Verification items for the finished model (mm, model axes). Face numbers are marked on the shaded views. Give positions to 0.01 mm unless a question says otherwise; leave off trailing zeros. Write each loop counter-clockwise with the first axis right and the second up, starting at its lowest first coordinate (ties: lowest second). Pieces come first, ordered by that corner, then holes.
from build123d import *

# Parameters (mm, degrees)
SKETCH1_W           = 188.724999994
SKETCH1_H           = 19.05
BOSS_EXTRUDE1_DEPTH = 109.3
HOLE1_D             = 3.175
HOLE1_DEPTH         = 31.75
HOLE1_CSINK_D       = 10.16
HOLE1_CSINK_ANGLE   = 82
HOLE1_TIP           = 0.953866233
HOLE2_D             = 3.175
HOLE2_DEPTH         = 31.75
HOLE2_CSINK_D       = 10.16
HOLE2_CSINK_ANGLE   = 82
HOLE2_TIP           = 0.953866233
HOLE3_D             = 3.175
HOLE3_DEPTH         = 31.75
HOLE3_CSINK_D       = 10.16
HOLE3_CSINK_ANGLE   = 82
HOLE3_TIP           = 0.953866233
HOLE4_D             = 63.5
HOLE4_DEPTH         = 19.05


with BuildPart() as part:
    # Sketch1 → Boss-Extrude1 (new body)
    with BuildSketch(Plane.XY):
        with Locations((-227.891965966, -292.321060846)):
            Rectangle(SKETCH1_W, SKETCH1_H)
    extrude(amount=BOSS_EXTRUDE1_DEPTH)

    # Hole1
    with Locations(Plane(origin=(-124.004465969, 10.424290059, -12.7), x_dir=(1, 0, 0), z_dir=(0, 0, -1))):
        with Locations((113.649999994, 128.807623392), (113.649999994, 23.940956725), (-94.599999994, 161.374290059), (94.599999994, 161.374290059), (0, 161.374290059), (0, 193.124290059), (0, 440.553783621), (0, 301.970350905), (40.979166666, 301.970350905), (166.795833328, 301.970350905), (207.774999994, 440.553783621), (207.774999994, 333.02141023), (207.774999994, 225.48903684), (207.774999994, 137.424290059), (207.774999994, 10.424290059), (-207.774999994, 10.424290059), (-207.774999994, 137.424290059), (-207.774999994, 225.48903684), (-207.774999994, 333.02141023), (-207.774999994, 440.553783621), (-166.795833328, 301.970350905), (-40.979166666, 301.970350905), (-113.649999994, 23.940956725), (-113.649999994, 128.807623392)):
            CounterSinkHole(HOLE1_D / 2, HOLE1_CSINK_D / 2, depth=HOLE1_DEPTH, counter_sink_angle=HOLE1_CSINK_ANGLE)
            with Locations((0, 0, -(HOLE1_DEPTH + HOLE1_TIP / 2))):  # 118° drill point
                Cone(0, HOLE1_D / 2, HOLE1_TIP, mode=Mode.SUBTRACT)

    # Hole2
    with Locations(Plane(origin=(-124.004465969, 10.424290059, 122), x_dir=(-1, 0, 0), z_dir=(0, 0, 1))):
        with Locations((113.649999994, 128.807623392), (113.649999994, 23.940956725), (-94.599999994, 161.374290059), (94.599999994, 161.374290059), (0, 161.374290059), (0, 193.124290059), (0, 440.553783621), (0, 301.970350905), (40.979166666, 301.970350905), (166.795833328, 301.970350905), (207.774999994, 440.553783621), (207.774999994, 333.02141023), (207.774999994, 225.48903684), (207.774999994, 137.424290059), (207.774999994, 10.424290059), (-207.774999994, 10.424290059), (-207.774999994, 137.424290059), (-207.774999994, 225.48903684), (-207.774999994, 333.02141023), (-207.774999994, 440.553783621), (-166.795833328, 301.970350905), (-40.979166666, 301.970350905), (-113.649999994, 23.940956725), (-113.649999994, 128.807623392)):
            CounterSinkHole(HOLE2_D / 2, HOLE2_CSINK_D / 2, depth=HOLE2_DEPTH, counter_sink_angle=HOLE2_CSINK_ANGLE)
            with Locations((0, 0, -(HOLE2_DEPTH + HOLE2_TIP / 2))):  # 118° drill point
                Cone(0, HOLE2_D / 2, HOLE2_TIP, mode=Mode.SUBTRACT)

    # Hole3
    with Locations(Plane(origin=(-124.004465969, 10.424290059, 122), x_dir=(-1, 0, 0), z_dir=(0, 0, 1))):
        with Locations((-207.774999994, 333.02141023), (-207.774999994, 225.48903684), (-207.774999994, 137.424290059), (-172.166666661, 4.074290059), (-146.083333327, 4.074290059), (-94.599999994, 161.374290059), (0, 161.374290059), (94.599999994, 161.374290059), (146.083333327, 4.074290059), (172.166666661, 4.074290059), (207.774999994, 137.424290059), (207.774999994, 225.48903684), (207.774999994, 333.02141023), (166.795833328, 301.970350905), (40.979166666, 301.970350905), (-40.979166666, 301.970350905), (-166.795833328, 301.970350905), (0, 193.124290059), (0, 301.970350905), (0, 412.366411751), (-126.349999994, 106.824290059), (-126.349999994, 58.624290059), (126.349999994, 58.624290059), (126.349999994, 106.824290059)):
            CounterSinkHole(HOLE3_D / 2, HOLE3_CSINK_D / 2, depth=HOLE3_DEPTH, counter_sink_angle=HOLE3_CSINK_ANGLE)
            with Locations((0, 0, -(HOLE3_DEPTH + HOLE3_TIP / 2))):  # 118° drill point
                Cone(0, HOLE3_D / 2, HOLE3_TIP, mode=Mode.SUBTRACT)

    # Hole4
    with Locations(Plane(origin=(0, -282.796060846, 0), x_dir=(1, 0, 0), z_dir=(0, 1, 0))):
        with Locations((-227.891965966, -54.65)):
            Hole(HOLE4_D / 2, depth=HOLE4_DEPTH)


solid = part.part
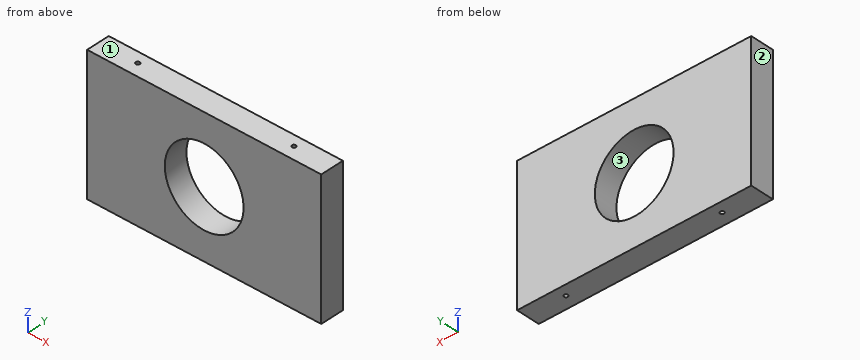
Item 1: Release check for a two-part mould opening along Z. For the marked faces 1, 2 and 3 record: released by +Z, released by -Z, zero draft, split by the parting line, or undercut.
Answer key:
face 1: released by +Z
face 2: zero draft
face 3: undercut
Item 2: Sectioned sample at A-A on z = 54.65. Record the cut outline in (x, y), then the cut area to 3 significant figures.
Answer key:
outline: (-322.25, -301.85) - (-259.64, -301.85) - (-259.64, -282.8) - (-322.25, -282.8) - close; (-196.14, -301.85) - (-133.53, -301.85) - (-133.53, -282.8) - (-196.14, -282.8) - close
area: 2,390 mm2
Item 3: Sectioned sample at C-C on z = 34.5. Record the cut outline in (x, y).
Answer key:
outline: (-322.25, -301.85) - (-252.43, -301.85) - (-252.43, -282.8) - (-322.25, -282.8) - close; (-203.36, -301.85) - (-133.53, -301.85) - (-133.53, -282.8) - (-203.36, -282.8) - close
Item 4: Sectioned sample at B-B on y = -295. Record the cut outline in (x, z).
Answer key:
outline: (-322.25, 0) - (-133.53, 0) - (-133.53, 109.3) - (-322.25, 109.3) - close; hole circle Ø63.5 at (-227.89, 54.65)
Item 5: Depth check by flat-ended pin: pin 1 (2.5 mm diameter, centred on x = -290.8, y = -291.55, fed in from +Z); pin 2 (3.5 mm diameter, centred on x = -290.8, y = -291.55, fed in from -Z); pin 3 (1.9 mm diameter, centred on x = -164.98, y = -291.55, fed in from +Z). Enter the tip coordinate at first touch or a pass-through.
Answer key:
pin 1: stops at z = 90.05
pin 2: stops at z = 0
pin 3: stops at z = 89.87
Item 6: Scan lines: line 1 along X through (y, z) = (-291.5, 16); line 2 along Z through (x, y) = (-204.5, -289.25); line 3 along X through (y, z) = (-290.5, 95). Record each from-to range of solid material in increasing order.
Answer key:
line 1: x = -322.25 to -292.39, -289.21 to -166.57, -163.4 to -133.53
line 2: z = 0 to 33.18, 76.12 to 109.3
line 3: x = -322.25 to -291.99, -289.61 to -166.18, -163.79 to -133.53
